from build123d import *

# Parameters (mm, degrees)
SKETCH1_W           = 55.5
SKETCH1_H           = 35
SKETCH1_W_2         = 45.5
SKETCH1_H_2         = 25
BOSS_EXTRUDE1_DEPTH = 28
SKETCH2_W           = 55.5
SKETCH2_H           = 35
BOSS_EXTRUDE2_DEPTH = 6
SKETCH4_R           = 1
CUT_EXTRUDE1_DEPTH  = 3.5
CUT_EXTRUDE2_REACH  = 47.481
SKETCH5_R           = 2
CUT_EXTRUDE3_REACH  = 45.131
SKETCH6_W           = 19.25
SKETCH6_H           = 22.5
CHAMFER1_SIZE       = 1.5
CUT_EXTRUDE4_REACH  = 45.131
SKETCH7_R           = 3
CHAMFER2_SIZE       = 1
SKETCH8_W           = 55.5
SKETCH8_H           = 9.5
BOSS_EXTRUDE3_DEPTH = 34
CUT_EXTRUDE5_REACH  = 53.527
SKETCH10_W          = 20
SKETCH10_H          = 7
SKETCH10_W_2        = 15
SKETCH10_H_2        = 4
CHAMFER7_SIZE       = 9
CHAMFER8_SIZE       = 5
CHAMFER9_SIZE       = 5
SKETCH12_R          = 1.45
CUT_EXTRUDE7_DEPTH  = 10
CUT_EXTRUDE8_REACH  = 57.806
SKETCH13_W          = 20
SKETCH13_H          = 25
CUT_EXTRUDE9_REACH  = 65.744
SKETCH14_W          = 25
SKETCH14_H          = 25
CHAMFER10_SIZE      = 5
CHAMFER11_SIZE      = 2
SKETCH15_R          = 2
CUT_EXTRUDE10_DEPTH = 5.2
CHAMFER12_SIZE      = 0.8


# Some blends are built 0.0001 mm under size
with BuildPart() as part:
    # Sketch1 → Boss-Extrude1 (new body)
    with BuildSketch(Plane(origin=(0, 0, 0), x_dir=(1, 0, 0), z_dir=(0, 1, 0))):
        Rectangle(SKETCH1_W, SKETCH1_H)
        Rectangle(SKETCH1_W_2, SKETCH1_H_2, mode=Mode.SUBTRACT)
    extrude(amount=BOSS_EXTRUDE1_DEPTH)

    # Sketch2 → Boss-Extrude2 (add)
    with BuildSketch(Plane.XZ):
        Rectangle(SKETCH2_W, SKETCH2_H)
    extrude(amount=BOSS_EXTRUDE2_DEPTH)

    # Sketch4 → Cut-Extrude1 (cut)
    with BuildSketch(Plane(origin=(0, 0, 0), x_dir=(1, 0, 0), z_dir=(0, 1, 0))):
        with Locations(Location((-4.2, 10.25, 0), (0, 0, 270))):
            Circle(SKETCH4_R)
        with Locations(Location((20.25, 10.25, 0), (0, 0, 270))):
            Circle(SKETCH4_R)
        with Locations(Location((20.25, -10.25, 0), (0, 0, 270))):
            Circle(SKETCH4_R)
        with Locations(Location((-4.2, -10.25, 0), (0, 0, 270))):
            Circle(SKETCH4_R)
    extrude(amount=-CUT_EXTRUDE1_DEPTH, mode=Mode.SUBTRACT)

    # Sketch5 → Cut-Extrude2 (cut, up to next)
    with BuildSketch(Plane(origin=(0, -3.5, 0), x_dir=(1, 0, 0), z_dir=(0, 1, 0)), mode=Mode.PRIVATE) as cut_extrude2_sk1:
        with Locations(Location((-4.2, 10.25, 0), (0, 0, 270))):
            Circle(SKETCH5_R)
    cut_extrude2_tool1 = extrude(cut_extrude2_sk1.sketch, amount=-CUT_EXTRUDE2_REACH, mode=Mode.PRIVATE) & part.part
    # Sketch5 → Cut-Extrude2 (cut, up to next)
    with BuildSketch(Plane(origin=(0, -3.5, 0), x_dir=(1, 0, 0), z_dir=(0, 1, 0)), mode=Mode.PRIVATE) as cut_extrude2_sk2:
        with Locations(Location((20.25, 10.25, 0), (0, 0, 270))):
            Circle(SKETCH5_R)
    cut_extrude2_tool2 = extrude(cut_extrude2_sk2.sketch, amount=-CUT_EXTRUDE2_REACH, mode=Mode.PRIVATE) & part.part
    # Sketch5 → Cut-Extrude2 (cut, up to next)
    with BuildSketch(Plane(origin=(0, -3.5, 0), x_dir=(1, 0, 0), z_dir=(0, 1, 0)), mode=Mode.PRIVATE) as cut_extrude2_sk3:
        with Locations(Location((20.25, -10.25, 0), (0, 0, 270))):
            Circle(SKETCH5_R)
    cut_extrude2_tool3 = extrude(cut_extrude2_sk3.sketch, amount=-CUT_EXTRUDE2_REACH, mode=Mode.PRIVATE) & part.part
    # Sketch5 → Cut-Extrude2 (cut, up to next)
    with BuildSketch(Plane(origin=(0, -3.5, 0), x_dir=(1, 0, 0), z_dir=(0, 1, 0)), mode=Mode.PRIVATE) as cut_extrude2_sk4:
        with Locations(Location((-4.2, -10.25, 0), (0, 0, 270))):
            Circle(SKETCH5_R)
    cut_extrude2_tool4 = extrude(cut_extrude2_sk4.sketch, amount=-CUT_EXTRUDE2_REACH, mode=Mode.PRIVATE) & part.part
    add(cut_extrude2_tool1.solids().sort_by_distance((-4.2, -3.5, -10.25))[0], mode=Mode.SUBTRACT)
    add(cut_extrude2_tool2.solids().sort_by_distance((20.25, -3.5, -10.25))[0], mode=Mode.SUBTRACT)
    add(cut_extrude2_tool3.solids().sort_by_distance((20.25, -3.5, 10.25))[0], mode=Mode.SUBTRACT)
    add(cut_extrude2_tool4.solids().sort_by_distance((-4.2, -3.5, 10.25))[0], mode=Mode.SUBTRACT)

    # Sketch6 → Cut-Extrude3 (cut, up to next)
    with BuildSketch(Plane(origin=(0, 0, 0), x_dir=(1, 0, 0), z_dir=(0, 1, 0)), mode=Mode.PRIVATE) as cut_extrude3_sk1:
        with Locations((7.875, 0)):
            Rectangle(SKETCH6_W, SKETCH6_H)
    cut_extrude3_tool1 = extrude(cut_extrude3_sk1.sketch, amount=-CUT_EXTRUDE3_REACH, mode=Mode.PRIVATE) & part.part
    add(cut_extrude3_tool1.solids().sort_by_distance((7.875, 0, 0))[0], mode=Mode.SUBTRACT)

    # Chamfer1
    chamfer1_edges = [part.edges().sort_by_distance(p)[0] for p in [
        (17.5, -3, -11.25),
        (17.5, -3, 11.25),
        (-1.75, -3, 11.25),
        (-1.75, -3, -11.25),
    ]]
    chamfer(chamfer1_edges, length=CHAMFER1_SIZE)

    # Sketch7 → Cut-Extrude4 (cut, up to next)
    with BuildSketch(Plane(origin=(0, 0, 0), x_dir=(1, 0, 0), z_dir=(0, 1, 0)), mode=Mode.PRIVATE) as cut_extrude4_sk1:
        with Locations(Location((-12.5, 0, 0), (0, 0, 270))):
            Circle(SKETCH7_R)
    cut_extrude4_tool1 = extrude(cut_extrude4_sk1.sketch, amount=-CUT_EXTRUDE4_REACH, mode=Mode.PRIVATE) & part.part
    add(cut_extrude4_tool1.solids().sort_by_distance((-12.5, 0, 0))[0], mode=Mode.SUBTRACT)

    # Chamfer2
    chamfer2_edges = [part.edges().sort_by_distance(p)[0] for p in [
        (-12.5, 0, -3),
        (-12.5, -6, -3),
    ]]
    chamfer(chamfer2_edges, length=CHAMFER2_SIZE)

    # Sketch8 → Boss-Extrude3 (add)
    with BuildSketch(Plane(origin=(0, 28, 0), x_dir=(1, 0, 0), z_dir=(0, 1, 0))):
        with Locations((0, -22.25)):
            Rectangle(SKETCH8_W, SKETCH8_H)
    boss_extrude3 = extrude(amount=-BOSS_EXTRUDE3_DEPTH)

    # Sketch10 → Cut-Extrude5 (cut, up to next)
    with BuildSketch(Plane(origin=(0, 28, 0), x_dir=(1, 0, 0), z_dir=(0, 1, 0)), mode=Mode.PRIVATE) as cut_extrude5_sk1:
        with Locations((0, -19.5)):
            Rectangle(SKETCH10_W, SKETCH10_H)
    cut_extrude5_tool1 = extrude(cut_extrude5_sk1.sketch, amount=-CUT_EXTRUDE5_REACH, mode=Mode.PRIVATE) & part.part
    # Sketch10 → Cut-Extrude5 (cut, up to next)
    with BuildSketch(Plane(origin=(0, 28, 0), x_dir=(1, 0, 0), z_dir=(0, 1, 0)), mode=Mode.PRIVATE) as cut_extrude5_sk2:
        with Locations((0, -25)):
            Rectangle(SKETCH10_W_2, SKETCH10_H_2)
    cut_extrude5_tool2 = extrude(cut_extrude5_sk2.sketch, amount=-CUT_EXTRUDE5_REACH, mode=Mode.PRIVATE) & part.part
    cut_extrude5_1 = cut_extrude5_tool1.solids().sort_by_distance((0, 28, 19.5))[0]
    add(cut_extrude5_1, mode=Mode.SUBTRACT)
    cut_extrude5_2 = cut_extrude5_tool2.solids().sort_by_distance((0, 28, 25))[0]
    add(cut_extrude5_2, mode=Mode.SUBTRACT)
    cut_extrude5 = cut_extrude5_1 + cut_extrude5_2  # Cut-Extrude5 as one shape, for the pattern or mirror that repeats it

    # Mirror3: Boss-Extrude3, Cut-Extrude5 across plane
    add(boss_extrude3.mirror(Plane.XY))
    add(cut_extrude5.mirror(Plane.XY), mode=Mode.SUBTRACT)

    # Chamfer7
    chamfer7_edges = [part.edges().sort_by_distance(p)[0] for p in [
        (17.625, -6, -27),
        (-27.75, 11, -27),
        (27.75, 11, -27),
        (-17.625, -6, -27),
        (17.625, -6, 27),
        (27.75, 11, 27),
        (-17.625, -6, 27),
        (-27.75, 11, 27),
    ]]
    chamfer(chamfer7_edges, length=CHAMFER7_SIZE)

    # Chamfer8
    chamfer8_edges = [part.edges().sort_by_distance(p)[0] for p in [
        (27.75, 28, 0),
        (-27.75, 28, 0),
    ]]
    chamfer(chamfer8_edges, length=CHAMFER8_SIZE - 0.0001)  # a hair under: the kernel refuses the full size

    # Chamfer9
    chamfer9_edges = [part.edges().sort_by_distance(p)[0] for p in [
        (27.75, -6, 0),
        (-27.75, -6, 0),
    ]]
    chamfer(chamfer9_edges, length=CHAMFER9_SIZE)

    # Sketch12 → Cut-Extrude7 (cut)
    with BuildSketch(Plane(origin=(0, 0, -27), x_dir=(-1, 0, 0), z_dir=(0, 0, -1))):
        with Locations((-14.375, 24)):
            Circle(SKETCH12_R)
        with Locations((14.375, 24)):
            Circle(SKETCH12_R)
        with Locations((14.375, 7)):
            Circle(SKETCH12_R)
        with Locations((-14.375, 7)):
            Circle(SKETCH12_R)
    cut_extrude7 = extrude(amount=-CUT_EXTRUDE7_DEPTH, mode=Mode.SUBTRACT)

    # Mirror4: Cut-Extrude7 across plane
    add(cut_extrude7.mirror(Plane.XY), mode=Mode.SUBTRACT)

    # Sketch13 → Cut-Extrude8 (cut, up to next)
    with BuildSketch(Plane.XY.offset(-12.5), mode=Mode.PRIVATE) as cut_extrude8_sk1:
        with Locations((0, 15.5)):
            Rectangle(SKETCH13_W, SKETCH13_H)
    cut_extrude8_tool1 = extrude(cut_extrude8_sk1.sketch, amount=-CUT_EXTRUDE8_REACH, mode=Mode.PRIVATE) & part.part
    cut_extrude8 = cut_extrude8_tool1.solids().sort_by_distance((0, 15.5, -12.5))[0]
    add(cut_extrude8, mode=Mode.SUBTRACT)

    # Sketch14 → Cut-Extrude9 (cut, up to next)
    with BuildSketch(Plane.ZY.offset(-22.75), mode=Mode.PRIVATE) as cut_extrude9_sk1:
        with Locations((0, 15.5)):
            Rectangle(SKETCH14_W, SKETCH14_H)
    cut_extrude9_tool1 = extrude(cut_extrude9_sk1.sketch, amount=-CUT_EXTRUDE9_REACH, mode=Mode.PRIVATE) & part.part
    cut_extrude9 = cut_extrude9_tool1.solids().sort_by_distance((22.75, 15.5, 0))[0]
    add(cut_extrude9, mode=Mode.SUBTRACT)

    # Mirror5: Cut-Extrude9 across plane
    add(cut_extrude9.mirror(Plane(origin=(0, 0, 0), x_dir=(0, 0, 1), z_dir=(1, 0, 0))), mode=Mode.SUBTRACT)

    # Mirror6: Cut-Extrude8 across plane
    add(cut_extrude8.mirror(Plane.XY), mode=Mode.SUBTRACT)

    # Chamfer10
    # the kernel refuses this chamfer: 5 mm, written as the material it adds along each edge
    with BuildSketch(Plane(origin=(-10, 3, -12.5), x_dir=(0.9996219169112968, -0.027495876610586403, 0), z_dir=(0, 0, -1)), Plane(origin=(10, 3, -12.5), x_dir=(0.027495876610586327, 0.9996219169112968, 0), z_dir=(0, 0, -1)), Plane(origin=(-10, 3, 12.5), x_dir=(-0.027495876610586317, 0.9996219169112968, 0), z_dir=(0, 0, 1))) as chamfer10_piece_1:
        Polygon((CHAMFER10_SIZE * 0.999621916911, -CHAMFER10_SIZE * 0.0274958766106), (-CHAMFER10_SIZE * 0.0274958766106, -CHAMFER10_SIZE * 0.999621916911), (0, 0), align=None)
    extrude(amount=3.5)
    with BuildSketch(Plane(origin=(22.75, 3, -12.5), x_dir=(0, -0.027495876610586403, 0.9996219169112968), z_dir=(1, 0, 0))) as chamfer10_piece_2:
        Polygon((CHAMFER10_SIZE * 0.999621916911, -CHAMFER10_SIZE * 0.0274958766106), (-CHAMFER10_SIZE * 0.0274958766106, -CHAMFER10_SIZE * 0.999621916911), (0, 0), align=None)
    extrude(amount=5)
    with BuildSketch(Plane(origin=(22.75, 3, 12.5), x_dir=(0, -0.027495876610586403, -0.9996219169112968), z_dir=(1, 0, 0)), Plane(origin=(-22.75, 3, -12.5), x_dir=(0, -0.027495876610586403, 0.9996219169112968), z_dir=(-1, 0, 0)), Plane(origin=(-22.75, 3, 12.5), x_dir=(0, 0.9996219169112968, 0.027495876610586327), z_dir=(-1, 0, 0))) as chamfer10_piece_3:
        Polygon((CHAMFER10_SIZE * 0.999621916911, CHAMFER10_SIZE * 0.0274958766106), (-CHAMFER10_SIZE * 0.0274958766106, CHAMFER10_SIZE * 0.999621916911), (0, 0), align=None)
    extrude(amount=5)
    with BuildSketch(Plane(origin=(10, 3, 12.5), x_dir=(0.027495876610586327, 0.9996219169112968, 0), z_dir=(0, 0, 1))) as chamfer10_piece_4:
        Polygon((CHAMFER10_SIZE * 0.999621916911, CHAMFER10_SIZE * 0.0274958766106), (-CHAMFER10_SIZE * 0.0274958766106, CHAMFER10_SIZE * 0.999621916911), (0, 0), align=None)
    extrude(amount=3.5)

    # Chamfer11
    chamfer11_edges = [part.edges().sort_by_distance(p)[0] for p in [
        (-10, 18, -12.5),
        (-10, 18, 12.5),
        (10, 18, 12.5),
        (10, 18, -12.5),
    ]]
    chamfer(chamfer11_edges, length=CHAMFER11_SIZE)

    # Sketch15 → Cut-Extrude10 (cut)
    with BuildSketch(Plane(origin=(0, 0, -27), x_dir=(-1, 0, 0), z_dir=(0, 0, -1))):
        with Locations((-14.375, 24)):
            Circle(SKETCH15_R)
        with Locations((14.375, 24)):
            Circle(SKETCH15_R)
        with Locations((14.375, 7)):
            Circle(SKETCH15_R)
        with Locations((-14.375, 7)):
            Circle(SKETCH15_R)
    cut_extrude10 = extrude(amount=-CUT_EXTRUDE10_DEPTH, mode=Mode.SUBTRACT)

    # Mirror7: Cut-Extrude10 across plane
    add(cut_extrude10.mirror(Plane.XY), mode=Mode.SUBTRACT)

    # Chamfer12
    chamfer12_edges = [part.edges().sort_by_distance(p)[0] for p in [
        (16.375, 7, -27),
        (-12.375, 7, -27),
        (-12.375, 24, -27),
        (16.375, 24, -27),
        (16.375, 7, 27),
        (-12.375, 7, 27),
        (-12.375, 24, 27),
        (16.375, 24, 27),
    ]]
    chamfer(chamfer12_edges, length=CHAMFER12_SIZE)


solid = part.part
CAD build for the part. Positions are in the model's coordinates, mm. A direction names the side the tool comes from. Coordinates: 2 decimals unless noted, no trailing zeros. Loops run counter-clockwise (first coordinate to the right, second up) from the corner with the lowest first, then second, coordinate; pieces in that order, holes last. Notation, with made-up numbers: (-12, -34.75) - (28, -34.75) arc R20 cw to (28, -5.75) - close; hole circle Ø6 at (73.25, 42). An arc over 180 degrees is marked (long way). Use one line per item in the form item = value. Start each with the question number.
1) Two-plate mould, pull along Z, no slides. Class faces 4 (the face through (-5.417, -4.732, -11.837)), 5 (the face through (-14, 24, 17)), 6 (the face through (-13, 25, -21.8)), 7 (the face through (17.5, -3, 0)): +Z half, -Z half, draft (parallel to the pull), parting line (faces both ways), or undercut.
2) Drill centre lines: L1, parallel to Z at x = 4, y = 1.5; L2, parallel to Z at x = -20.5, y = 18; L3, parallel to X at y = 25, z = 24. Where is each one in solid material? Low to high. Write a range as from..to.
3) Tool access for faces 1 (the face through (16.76, -2.96, -10.49)), 2 (the face through (13.5, 22.2, 24)), 3 (the face through (13, 25, -21.8)): list every direction of +Z, -Z, +X, -X, +Y, -Y with a clear straight run to the whole face (end or side of a thin tool).
4) Band-saw the part on B-B (x = -4.2). Give the cut face in (y, z).
5) Band-saw the part on A-A (z = 0). Give the cut face in (x, y), and give its area (4 significant figures).
6) Band-saw the part on C-C (z = 6.5). Give the cut face in (x, y).
7) Flat gauge pins, fed straight in: pin 1 (6.5 mm diameter, centred on x = -4.2, z = -10.25, fed in from +Y); pin 2 (2 mm diameter, centred on x = -14, y = 24, fed in from +Z); pin 3 (4.5 mm diameter, centred on y = 20, z = 25, fed in from -X). Where does each tip first touch, or does it go through?
8) Band-saw the part on D-D (y = 17). State how many separate pieces and enclosed holes the cut face has, and give its area (4 significant figures).
Check values:
q1.face_4 = undercut
q1.face_5 = +Z half
q1.face_6 = -Z half
q1.face_7 = undercut
q2.L1 = -16..-12.5, 12.5..16
q2.L2 = -25.25..-12.5, 12.5..25.25
q2.L3 = -21.75..-16.11, -12.64..-7.5, 7.5..12.64, 16.11..21.75
q3.face_1 = +Y, -Y
q3.face_2 = +Z
q3.face_3 = -Z
q4.outline = (-6, -16) - (3, -16) - (3, -12.5) - (0, -12.5) - (0, -11.25) - (-3.5, -11.25) - (-3.5, -12.25) - (-6, -12.25) - close; (-6, -8.25) - (-3.5, -8.25) - (-3.5, -9.25) - (0, -9.25) - (0, 9.25) - (-3.5, 9.25) - (-3.5, 8.25) - (-6, 8.25) - close; (-6, 12.25) - (-3.5, 12.25) - (-3.5, 11.25) - (0, 11.25) - (0, 12.5) - (3, 12.5) - (3, 16) - (-6, 16) - close
q5.outline = (-27.75, -1) - (-22.75, -6) - (-16.5, -6) - (-15.5, -5) - (-15.5, -1) - (-16.5, 0) - (-22.75, 0) - (-22.75, 3) - (-27.75, 3) - close; (-9.5, -5) - (-8.5, -6) - (-1.75, -6) - (-1.75, 0) - (-8.5, 0) - (-9.5, -1) - close; (17.5, -6) - (22.75, -6) - (27.75, -1) - (27.75, 3) - (22.75, 3) - (22.75, 0) - (17.5, 0) - close
q5.area = 184.5 mm2
q6.outline = (-27.75, -1) - (-22.75, -6) - (-1.75, -6) - (-1.75, 0) - (-22.75, 0) - (-22.75, 3) - (-27.75, 3) - close; (17.5, -6) - (22.75, -6) - (27.75, -1) - (27.75, 3) - (22.75, 3) - (22.75, 0) - (17.5, 0) - close
q7.pin_1 = 4.55
q7.pin_2 = 17
q7.pin_3 = -23
q8.separate_pieces = 4
q8.enclosed_holes = 0
q8.area = 899.5 mm2
